from build123d import *

# Parameters (mm, degrees)
SKETCH1_R           = 1.8
BOSS_EXTRUDE1_DEPTH = 1.5
CHAMFER1_SIZE       = 0.15


with BuildPart() as part:
    # Sketch1 → Boss-Extrude1 (new, symmetric)
    with BuildSketch(Plane(origin=(0, 0, 0), x_dir=(1, 0, 0), z_dir=(0, 1, 0))):
        Polygon((0, 3.914434825), (-3.39, 1.957217413), (-3.39, -1.957217413), (0, -3.914434825), (3.39, -1.957217413), (3.39, 1.957217413), align=None)
        with Locations(Location((0, 0, 0), (0, 0, 270))):
            Circle(SKETCH1_R, mode=Mode.SUBTRACT)
    extrude(amount=BOSS_EXTRUDE1_DEPTH, both=True)

    # Chamfer1
    chamfer1_edges = [part.edges().sort_by_distance(p)[0] for p in [
        (0, -1.5, -1.8),
        (0, 1.5, -1.8),
    ]]
    chamfer(chamfer1_edges, length=CHAMFER1_SIZE)

    # Sketch2 → Cut-Revolve1 (revolve, cut)
    with BuildSketch(Plane.XY):
        Polygon((-3.39, 1.5), (-5, 0.74924467), (-5, 1.5), align=None)
    cut_revolve1 = revolve(axis=Axis((0, 0, 0), (0, 1, 0)), mode=Mode.SUBTRACT)

    # Mirror1: Cut-Revolve1 across plane
    add(cut_revolve1.mirror(Plane.ZX), mode=Mode.SUBTRACT)


solid = part.part
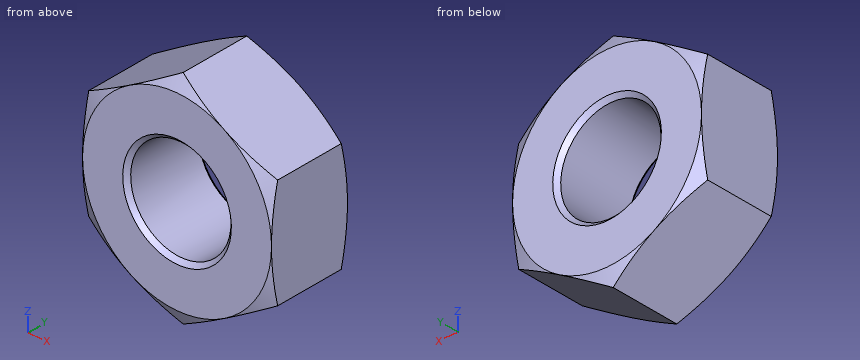
Source: CAD feature listing. Evaluate the final solid. Frame: model axes, mm. Round coordinates to 2 decimals unless told otherwise and drop trailing zeros. Write each loop counter-clockwise with the first axis right and the second up, starting at its lowest first coordinate (ties: lowest second). Pieces come first, ordered by that corner, then holes. Notation, with made-up numbers: M 64,48 L 71,48 A19 cw 71,60 Z; hole C -3,54 d4. An arc over 180 degrees is marked long. One line per item, written item: value. Start each with the question number.
Item 1: Pin query (flat end, axial travel): pin 1 (1 mm diameter, centred on x = 0, z = -1, fed in from +Y). Return the tip coordinate at first contact, or that it passes through.
Item 2: Section query A-A (y = 0.75). Return the cut outline in (x, z).
Item 3: Ray query, L1, parallel to X at y = -0.55, z = 0; L2, parallel to Z at x = -1.5, y = 1.1; L3, parallel to X at y = 0.45, z = 1.5. Return the intervals inside material, ascending. Write a range as from..to.
Result set:
1. pin 1: passes through
2. outline: M -3.39,-1.96 L 0,-3.91 L 3.39,-1.96 L 3.39,1.96 L 0,3.91 L -3.39,1.96 Z; hole C 0,0 d3.6
3. L1: x = -3.39..-1.8, 1.8..3.39
3. L2: z = -3.05..-0.99, 0.99..3.05
3. L3: x = -3.39..-0.99, 0.99..3.39
